Autodesk Inventor part; units mm, degrees
ref_plane "YZ Plane" through (0, 0, 0) normal (1, 0, 0) x (0, 1, 0)
ref_plane "XZ Plane" through (0, 0, 0) normal (0, 1, 0) x (-1, 0, 0)
ref_plane "XY Plane" through (0, 0, 0) normal (0, 0, 1) x (1, 0, 0)
sketch "Sketch1" plane through (0, 0, 0) normal (0, 0, 1) x (1, 0, 0)
  line L0 (0, 0) -> (250, 0)
  line L1 (250, 0) -> (250, 35)
  line L2 (250, 35) -> (0, 35)
  line L3 (0, 35) -> (0, 0)
  line L4 (25, 35) -> (25, 0)
  line L5 (3.9, 8.9) -> (46.1, 8.9)
  line L6 (46.1, 8.9) -> (46.1, 26.1)
  line L7 (46.1, 26.1) -> (3.9, 26.1)
  line L8 (3.9, 26.1) -> (3.9, 8.9)
  line L9 (3.9, 8.9) -> (46.1, 26.1) construction
  line L10 (46.1, 8.9) -> (3.9, 26.1) construction
  circle A0 centre (3.9, 26.1) radius 2.5
  circle A1 centre (46.1, 26.1) radius 2.5
  circle A2 centre (3.9, 8.9) radius 2.5
  circle A3 centre (46.1, 8.9) radius 2.5
  circle A4 centre (3.9, 26.1) radius 0.6
  circle A5 centre (46.1, 26.1) radius 0.6
  circle A6 centre (3.9, 8.9) radius 0.6
  circle A7 centre (46.1, 8.9) radius 0.6
  line L11 (125, 35) -> (125, 0)
  line L12 (225, 35) -> (225, 0)
  line L13 (246.1, 8.9) -> (203.9, 8.9)
  line L14 (203.9, 8.9) -> (203.9, 26.1)
  line L15 (203.9, 26.1) -> (246.1, 26.1)
  line L16 (246.1, 26.1) -> (246.1, 8.9)
  line L17 (246.1, 8.9) -> (203.9, 26.1) construction
  line L18 (203.9, 8.9) -> (246.1, 26.1) construction
  circle A8 centre (246.1, 26.1) radius 2.5
  circle A9 centre (203.9, 26.1) radius 2.5
  circle A10 centre (246.1, 8.9) radius 2.5
  circle A11 centre (203.9, 8.9) radius 2.5
  circle A12 centre (246.1, 26.1) radius 0.6
  circle A13 centre (203.9, 26.1) radius 0.6
  circle A14 centre (246.1, 8.9) radius 0.6
  circle A15 centre (203.9, 8.9) radius 0.6
  line L19 (17.5, 7) -> (32.5, 7)
  line L20 (32.5, 7) -> (32.5, 28)
  line L21 (32.5, 28) -> (17.5, 28)
  line L22 (17.5, 28) -> (17.5, 7)
  line L23 (17.5, 7) -> (32.5, 28) construction
  line L24 (32.5, 7) -> (17.5, 28) construction
  line L25 (46.1, 26.1) -> (3.9, 26.1)
  line L26 (232.5, 7) -> (217.5, 7)
  line L27 (217.5, 7) -> (217.5, 28)
  line L28 (217.5, 28) -> (232.5, 28)
  line L29 (232.5, 28) -> (232.5, 7)
  point P0 (25, 17.5)
  point P1 (225, 17.5)
  point P2 (6.4, 26.1)
  point P3 (17.5, 26.1)
  point P4 (32.5, 26.1)
  point P5 (43.6, 26.1)
  point P6 (46.1, 23.6)
  point P7 (46.1, 11.4)
  point P8 (43.6, 8.9)
  point P9 (32.5, 8.9)
  point P10 (17.5, 8.9)
  point P11 (6.4, 8.9)
  point P12 (3.9, 11.4)
  point P13 (3.9, 23.6)
  point P14 (217.5, 8.9)
  point P15 (206.4, 8.9)
  point P16 (203.9, 11.4)
  point P17 (203.9, 23.6)
  point P18 (206.4, 26.1)
  point P19 (217.5, 26.1)
  point P20 (232.5, 26.1)
  point P21 (243.6, 26.1)
  point P22 (246.1, 23.6)
  point P23 (246.1, 11.4)
  point P24 (243.6, 8.9)
  point P25 (232.5, 8.9)
  dimension "d0" = 250
  dimension "d1" = 35
  dimension "d2" = 17.2
  dimension "d3" = 42.2
  dimension "d4" = 5
  dimension "d5" = 5
  dimension "d6" = 5
  dimension "d7" = 5
  dimension "d8" = 1.2
  dimension "d9" = 1.2
  dimension "d10" = 1.2
  dimension "d11" = 1.2
  dimension "d12" = 25
  dimension "d13" = 15
  dimension "d14" = 21
extrude "Extrusion1" add sketch "Sketch1" along normal blind 5.5 contours L3 L2 L4 L21 L22 L7 A0 L8 A2 L5 L19 L0 | L4 L19 L20 L5 A3 L6 A1 L7 L21 L2 L11 L0 | L11 L2 L12 L28 L27 L15 A9 L14 A11 L13 L26 L0 | L12 L26 L29 L13 A10 L16 A8 L15 L28 L2 L1 L0 | A2 L8 A6 L5 | L5 A6 L8 A2 | A3 L6 A7 L5 | L5 A7 L6 A3 | A1 L6 A5 L7 | L7 A5 L6 A1 | A0 L8 A4 L7 | L7 A4 L8 A0 | A6 L8 L5 | L5 L8 A6 | A7 L6 L5 | L5 L6 A7 | A10 L16 A14 L13 | L13 A14 L16 A10 | A11 L14 A15 L13 | L13 A15 L14 A11 | A5 L6 L7 | L7 L6 A5 | A4 L8 L7 | L7 L8 A4 | A9 L14 A13 L15 | L15 A13 L14 A9 | A8 L16 A12 L15 | L15 A12 L16 A8 | A14 L16 L13 | L13 L16 A14 | A15 L14 L13 | L13 L14 A15 | A13 L14 L15 | L15 L14 A13 | A12 L16 L15 | L15 L16 A12
extrude "Extrusion2" cut sketch "Sketch1" along normal blind 5.5 contours A6 L8 L5 | L5 L8 A6 | A7 L6 L5 | L5 L6 A7 | A5 L6 L7 | L7 L6 A5 | A4 L8 L7 | L7 L8 A4 | A14 L16 L13 | L13 L16 A14 | A15 L14 L13 | L13 L14 A15 | A13 L14 L15 | L15 L14 A13 | A12 L16 L15 | L15 L16 A12
sketch "Sketch2" plane through (0, 0, 5.5) normal (0, 0, 1) x (1, 0, 0)
  line L0 (200, -30) -> (50, -30)
  line L1 (50, -30) -> (50, 30)
  line L2 (50, 30) -> (200, 30)
  line L3 (200, 30) -> (200, -30)
  line L4 (0, 0) -> (250, 0)
  line L5 (200, -30) -> (50, 30) construction
  line L6 (50, -30) -> (200, 30) construction
  point P0 (125, 0)
  point P1 (50, 0)
  point P2 (200, 0)
  dimension "d19" = 150
  dimension "d20" = 60
extrude "Extrusion3" cut sketch "Sketch2" against normal blind 5.5 contours L4 L1 L2 L3
sketch "Sketch3" plane through (0, 0, 5.5) normal (0, 0, 1) x (1, 0, 0)
  line L0 (50, 30) -> (200, 30)
  line L1 (105, 30) -> (145, 30)
  line L2 (145, 30) -> (145, 35)
  line L3 (145, 35) -> (105, 35)
  line L4 (105, 35) -> (105, 30)
  point P0 (0, 0)
  point P1 (145, 30)
  dimension "d23" = 40
  dimension "d24" = 5
  dimension "d25" = 55
extrude "Extrusion4" add sketch "Sketch3" along normal blind 10
sketch "Sketch4" plane through (105, 35, 5.5) normal (0, 1, 0) x (-1, 0, 0)
  line L0 (0, 10) -> (-40, 10)
  line L1 (-20, 10) -> (-20, 0)
  line L2 (-145, 0) -> (105, 0)
  circle A0 centre (-10, 5) radius 1.5
  circle A1 centre (-30, 5) radius 1.5
  line L3 (-10, 5) -> (-30, 5)
  point P0 (105, -5.5)
  dimension "d28" = 10
  dimension "d29" = 3
  dimension "d30" = 3
  dimension "d31" = 10
extrude "Extrusion5" cut sketch "Sketch4" against normal blind 10
fillet "Fillet1" radius 10 8 edges at (0, 35, 2.75) (50, 0, 2.75) (0, 0, 2.75) (145, 32.5, 15.5) (105, 32.5, 15.5) (200, 0, 2.75) (250, 0, 2.75) (250, 35, 2.75)
sketch "Sketch5" plane through (0, 0, 5.5) normal (0, 0, 1) x (1, 0, 0)
  arc A0 (40, 0) -> (50, 10) centre (40, 10) ccw
  line L0 (50, 10) -> (86.2042, 30)
  line L1 (50, 30) -> (105, 30)
  line L2 (50, 10) -> (50, 30)
  line L3 (50, 13.4273) -> (80, 30)
  arc A1 (0, 10) -> (10, 0) centre (10, 10) ccw
  line L4 (10, 0) -> (40, 0)
  arc A2 (40, 0) -> (50, 10) centre (40, 10) ccw
  line L5 (50, 10) -> (50, 30)
  line L6 (50, 30) -> (105, 30)
  line L7 (105, 30) -> (105, 35)
  line L8 (105, 35) -> (10, 35)
  arc A3 (10, 35) -> (0, 25) centre (10, 25) ccw
  line L9 (0, 25) -> (0, 10)
  circle A4 centre (46.1, 8.9) radius 0.6
  circle A5 centre (3.9, 8.9) radius 0.6
  circle A6 centre (46.1, 26.1) radius 0.6
  circle A7 centre (3.9, 26.1) radius 0.6
  line L10 (6.4, 26.1) -> (17.5, 26.1)
  line L11 (17.5, 26.1) -> (17.5, 28)
  line L12 (17.5, 28) -> (32.5, 28)
  line L13 (32.5, 28) -> (32.5, 26.1)
  line L14 (32.5, 26.1) -> (43.6, 26.1)
  arc A8 (43.6, 26.1) -> (46.1, 23.6) centre (46.1, 26.1) ccw
  line L15 (46.1, 23.6) -> (46.1, 11.4)
  arc A9 (46.1, 11.4) -> (43.6, 8.9) centre (46.1, 8.9) ccw
  line L16 (43.6, 8.9) -> (32.5, 8.9)
  line L17 (32.5, 8.9) -> (32.5, 7)
  line L18 (32.5, 7) -> (17.5, 7)
  line L19 (17.5, 7) -> (17.5, 8.9)
  line L20 (17.5, 8.9) -> (6.4, 8.9)
  arc A10 (6.4, 8.9) -> (3.9, 11.4) centre (3.9, 8.9) ccw
  line L21 (3.9, 11.4) -> (3.9, 23.6)
  arc A11 (3.9, 23.6) -> (6.4, 26.1) centre (3.9, 26.1) ccw
  point P0 (0, 0)
  dimension "d35" = 3
  dimension "d36" = 30
extrude "Extrusion6" add sketch "Sketch5" against normal blind 5.5 contours L2 L3 L1 L0
ref_plane "Work Plane1" through (125, 30, 5.5) normal (1, 0, 0) x (0, 0, -1)
mirror "Mirror1" about plane through (125, 30, 5.5) normal (1, 0, 0) of "Extrusion6"
properties part number "UltrasonicHolder"
CAD build for the part. Positions are in the model's coordinates, mm. A direction names the side the tool comes from. Coordinates: 2 decimals unless noted, no trailing zeros. Order: outer loops, then holes, each group sorted by start corner. A loop starts at its lowest first (then second) coordinate and runs counter-clockwise, first axis right, second up. Notation, with made-up numbers: (54.25, 32) -> (67.25, 32) arc R11 ccw to (67.25, 37) -> close; hole circle Ø6 at (27.5, 69.5). An arc over 180 degrees is marked (long way). Use one line per item in the form item = value. Start each with the question number.
1) Band-saw the part on A-A on x = 186. Give the cut face in (y, z).
2) Band-saw the part on B-B on y = 18.5. Give the cut face in (x, z).
3) Band-saw the part on C-C on z = 3. State how many separate pieces and enclosed holes the cut face has, then the cut area to 3 significant figures.
4) Drop flat-ended pins along their axis: pin 1 (0.7 mm diameter, centred on x = 46.1, y = 8.9, fed in from -Z); pin 2 (1 mm diameter, centred on x = 70.5, y = 31, fed in from +Z); pin 3 (1.5 mm diameter, centred on y = 8, z = 2, fed in from -X). Give the stop position or say it passes through.
5) Tool access for faces 4 (the flat face through (124, 30, 6)), 5 (the flat face through (41, 27, 5.5)), 6 (the flat face through (38, 26.1, 3)): list every direction of +Z, -Z, +X, -X, +Y, -Y with a clear straight run to the whole face (end or side of a thin tool).
6) Drill centre lines: L1, parallel to Y at x = 15, z = 2.25; L2, parallel to X at y = 27.5, z = 0.5; L3, parallel to Y at x = 128, z = 3.25. Where is each one in solid material? Low to high. Write a range as [from, to].
7) Pull direction Y, two halves, no side cores. Call faces 1 (the cylindrical face through (2.85, 3.01, 2.79)), 2 (the flat face through (25, 28, 3)), 3 (the flat face through (125, 33, 15.5)): +Y half, -Y half, draft (parallel to the pull), parting line (faces both ways), or undercut.
Entries:
q1.outline = (17.73, 0) -> (21.16, 0) -> (21.16, 5.5) -> (17.73, 5.5) -> close; (30, 0) -> (35, 0) -> (35, 5.5) -> (30, 5.5) -> close
q2.outline = (0, 0) -> (3.9, 0) -> (3.9, 5.5) -> (0, 5.5) -> close; (46.1, 0) -> (50, 0) -> (50, 5.5) -> (46.1, 5.5) -> close; (59.18, 0) -> (65.39, 0) -> (65.39, 5.5) -> (59.18, 5.5) -> close; (184.61, 0) -> (190.82, 0) -> (190.82, 5.5) -> (184.61, 5.5) -> close; (200, 0) -> (203.9, 0) -> (203.9, 5.5) -> (200, 5.5) -> close; (246.1, 0) -> (250, 0) -> (250, 5.5) -> (246.1, 5.5) -> close
q3.separate_pieces = 1
q3.enclosed_holes = 12
q3.area = 2,810 mm2
q4.pin_1 = through
q4.pin_2 = 5.5
q4.pin_3 = 0.08
q5.face_4 = +Z, -Z, -Y
q5.face_5 = +Z, -X, +Y, -Y
q5.face_6 = +Z, -Z
q6.L1 = [0, 8.9], [26.1, 35]
q6.L2 = [0.32, 17.5], [32.5, 50], [75.47, 81.68], [168.32, 174.53], [200, 217.5], [232.5, 249.68]
q6.L3 = [30, 35]
q7.face_1 = -Y half
q7.face_2 = undercut
q7.face_3 = draft
